Can you work these out from the model? Positions are in its coordinate system, mm. A direction names the side the tool comes from. Give positions to 0.01 mm unless a question says otherwise; leave off trailing zeros. Loops run counter-clockwise (first coordinate to the right, second up) from the corner with the lowest first, then second, coordinate; pieces in that order, holes last. Notation, with made-up numbers: (50.25, 53) - (108.25, 53) arc R8 cw to (108.25, 60) - close; hole circle Ø9 at (41.5, 86). An arc over 180 degrees is marked (long way). Answer as a JSON object with one key per item and string values. Group by question number.
Item 1: Suppose I cut it at C-C on z = 28. Write out the boundary of the cut face in (x, y).
Item 2: Will these pins go through, and if not, where does the flat tip stop? pin 1 (2 mm diameter, centred on y = 111, z = 27, fed in from +X); pin 2 (2 mm diameter, centred on y = 151.5, z = 27.5, fed in from +X); pin 3 (1.2 mm diameter, centred on y = 107.5, z = 27.5, fed in from -X).
Item 3: Thinking about a two-plate mould opening in X: for faces 1 (the cylindrical face through (43, 41.64, 27.68)), 2 (the cylindrical face through (-36.126, 145.388, 27.678)), 3 (the cylindrical face through (53.2, 61.81, 27.68)), which applies, pulls with the +X half, pulls with the -X half, needs draft (parallel to the pull), parting line crosses it, or undercut?
Item 4: Suppose I cut it at A-A on y = 187.2. Write out the boundary of the cut face in (x, z), and give its area (3 significant figures).
Item 5: Suppose I cut it at B-B on x = 39.65. Write out the boundary of the cut face in (y, z).
Item 6: Please list where these lines run through material, in increasing order: L1, parallel to X at y = 46, z = 27; L2, parallel to Y at x = 39.65, z = 27.25; L3, parallel to Y at x = 38, z = 28.4.
Item 7: Suppose I cut it at D-D on y = 106.5. Write out the boundary of the cut face in (x, z).
Item 8: Which directions (+Z, -Z, +X, -X, +Y, -Y) give clear straight access to the entire face, cutting with the end or side of a thin tool? Please do faces 4 (the flat face through (-35.65, 116, 28)), 5 (the cylindrical face through (36.126, 145.388, 27.678)), 6 (the flat face through (-1, 203.2, 28)).
from build123d import *

# Parameters (mm, degrees)
SKETCH12_W                     = 4.57134
SKETCH12_H                     = 203.2
BOSS_EXTRUDE1_START            = -173.2
BOSS_EXTRUDE1_DEPTH            = 173.2
BOSS_EXTRUDE2_DEPTH            = 4
SKETCH29_W                     = 5.5
SKETCH29_H                     = 4
M10_CLEARANCE_HOLE1_AT_2_COUNT = 2
M10_CLEARANCE_HOLE1_AT_2_PITCH = 141.2
FILLET1_R                      = 10
MIRROR1_COPY_1_SKETCH_W        = 5.5
MIRROR1_COPY_1_SKETCH_H        = 4
FILLET1_OF_MIRROR1_R           = 10


with BuildPart() as part:
    # Sketch12 → Revolve1 (revolve)
    with BuildSketch(Plane.XY, mode=Mode.PRIVATE) as revolve1_sk:
        with Locations((-23.36433, 101.6)):
            Rectangle(SKETCH12_W, SKETCH12_H)
    revolve(revolve1_sk.sketch.rotate(Axis((0, 0, 0), (0, 1, 0)), 270), axis=Axis((0, 0, 0), (0, 1, 0)))

    # Sketch14 → Boss-Extrude1 (add)
    with BuildSketch(Plane(origin=(0, 30, 0), x_dir=(-1, 0, 0), z_dir=(0, -1, 0)).offset(BOSS_EXTRUDE1_START)):
        with BuildLine():
            Line((-25.65, 0), (-25.65, -25.65))
            Line((-25.65, -25.65), (1.5e-08, -25.65))
            ThreePointArc((1.5e-08, -25.65), (-18.137288932, -18.137288943), (-25.65, 0))
        make_face()
        with BuildLine():
            ThreePointArc((25.65, 0), (18.137288943, -18.137288932), (1.5e-08, -25.65))
            Line((1.5e-08, -25.65), (25.65, -25.65))
            Line((25.65, -25.65), (25.65, 0))
        make_face()
    extrude(amount=BOSS_EXTRUDE1_DEPTH)


with BuildPart() as body_2:
    # Sketch27 → Boss-Extrude2 (new body)
    with BuildSketch(Plane.XY.offset(25.65)):
        Polygon((53.65, 203.2), (-25.65, 203.2), (-25.65, 30), (53.65, 30), (53.65, 62), (35.65, 87.706664121), (35.65, 145.493335879), (53.65, 171.2), align=None)
    boss_extrude2 = extrude(amount=BOSS_EXTRUDE2_DEPTH)

    # Sketch29 → M10 Clearance Hole1 (revolve, cut)
    with BuildSketch(Plane(origin=(39.65, 46, 25.65), x_dir=(0, 1, 0), z_dir=(1, 0, 0))):
        with Locations((2.75, 2)):
            Rectangle(SKETCH29_W, SKETCH29_H)
    m10_clearance_hole1 = revolve(axis=Axis((39.65, 46, 19.3), (0, 0, 1)), mode=Mode.SUBTRACT)

    # M10 Clearance Hole1 at 2: M10 Clearance Hole1 ×2
    with Locations(*[(0, i * M10_CLEARANCE_HOLE1_AT_2_PITCH, 0) for i in range(1, M10_CLEARANCE_HOLE1_AT_2_COUNT)]):
        add(m10_clearance_hole1, mode=Mode.SUBTRACT)

    # Fillet1
    fillet1_edges = [body_2.edges().sort_by_distance(p)[0] for p in [
        (53.65, 203.2, 27.65),
        (53.65, 171.2, 27.65),
        (35.65, 145.493335879, 27.65),
        (35.65, 87.706664121, 27.65),
        (53.65, 62, 27.65),
        (53.65, 30, 27.65),
    ]]
    fillet(fillet1_edges, radius=FILLET1_R)

    # Mirror1: Boss-Extrude2, M10 Clearance Hole1 across plane
    add(boss_extrude2.mirror(Plane(origin=(0, 0, 0), x_dir=(0, 0, 1), z_dir=(1, 0, 0))))
    add(m10_clearance_hole1.mirror(Plane(origin=(0, 0, 0), x_dir=(0, 0, 1), z_dir=(1, 0, 0))), mode=Mode.SUBTRACT)

    # Mirror1 copy 1 sketch → Mirror1 copy 1 (revolve, cut)
    with BuildSketch(Plane(origin=(-39.65, 187.2, 25.65), x_dir=(0, 1, 0), z_dir=(-1, 0, 0))):
        with Locations((2.75, -2)):
            Rectangle(MIRROR1_COPY_1_SKETCH_W, MIRROR1_COPY_1_SKETCH_H)
    revolve(axis=Axis((-39.65, 187.2, 19.3), (0, 0, -1)), mode=Mode.SUBTRACT)

    # Fillet1 of Mirror1
    fillet1_of_mirror1_edges = [body_2.edges().sort_by_distance(p)[0] for p in [
        (-53.65, 203.2, 27.65),
        (-53.65, 171.2, 27.65),
        (-35.65, 145.493335879, 27.65),
        (-35.65, 87.706664121, 27.65),
        (-53.65, 62, 27.65),
        (-53.65, 30, 27.65),
    ]]
    fillet(fillet1_of_mirror1_edges, radius=FILLET1_OF_MIRROR1_R)


solid = body_2.part
Worked out:
{
 "1": {"outline": "(-53.65, 40) arc R10 ccw to (-43.65, 30) - (43.65, 30) arc R10 ccw to (53.65, 40) - (53.65, 58.85) arc R10 ccw to (51.84, 64.58) - (37.46, 85.12) arc R10 cw to (35.65, 90.86) - (35.65, 142.34) arc R10 cw to (37.46, 148.08) - (51.84, 168.62) arc R10 ccw to (53.65, 174.35) - (53.65, 193.2) arc R10 ccw to (43.65, 203.2) - (-43.65, 203.2) arc R10 ccw to (-53.65, 193.2) - (-53.65, 174.35) arc R10 ccw to (-51.84, 168.62) - (-37.46, 148.08) arc R10 cw to (-35.65, 142.34) - (-35.65, 90.86) arc R10 cw to (-37.46, 85.12) - (-51.84, 64.58) arc R10 ccw to (-53.65, 58.85) - close; hole circle Ø11 at (-39.65, 46); hole circle Ø11 at (-39.65, 187.2); hole circle Ø11 at (39.65, 46); hole circle Ø11 at (39.65, 187.2)"},
 "2": {"pin 1": "stops at x = 35.65", "pin 2": "stops at x = 40.56", "pin 3": "stops at x = -35.65"},
 "3": {"face 1": "undercut", "face 2": "pulls with the -X half", "face 3": "pulls with the +X half"},
 "4": {"outline": "(-53.65, 25.65) - (-45.15, 25.65) - (-45.15, 29.65) - (-53.65, 29.65) - close; (-34.15, 25.65) - (34.15, 25.65) - (34.15, 29.65) - (-34.15, 29.65) - close; (45.15, 25.65) - (53.65, 25.65) - (53.65, 29.65) - (45.15, 29.65) - close", "area": "341 mm2"},
 "5": {"outline": "(30, 25.65) - (40.5, 25.65) - (40.5, 29.65) - (30, 29.65) - close; (51.5, 25.65) - (81.99, 25.65) - (81.99, 29.65) - (51.5, 29.65) - close; (151.21, 25.65) - (181.7, 25.65) - (181.7, 29.65) - (151.21, 29.65) - close; (192.7, 25.65) - (203.2, 25.65) - (203.2, 29.65) - (192.7, 29.65) - close"},
 "6": {"L1": "x = -53.65 to -45.15, -34.15 to 34.15, 45.15 to 53.65", "L2": "y = 30 to 40.5, 51.5 to 81.99, 151.21 to 181.7, 192.7 to 203.2", "L3": "y = 30 to 40.75, 51.25 to 84.35, 148.85 to 181.95, 192.45 to 203.2"},
 "7": {"outline": "(-35.65, 25.65) - (35.65, 25.65) - (35.65, 29.65) - (-35.65, 29.65) - close"},
 "8": {"face 4": "+Z, -Z, -X", "face 5": "+Z, -Z, +X", "face 6": "+Z, -Z, +X, -X, +Y"}
}
